from build123d import *

# Parameters (mm, degrees)
F0_R     = 15
F1_DEPTH = 25
F2_START = 25
F0_R_2   = 3
F2_DEPTH = 10
F3_R     = 10.8639610307
F4_R     = 5


with BuildPart() as f1:
    # F0 (on Top) → F1 (new body)
    with BuildSketch(Plane.XY):
        Circle(F0_R)
        Polygon((12.5, 0), (6.25, -10.8253175473), (-6.25, -10.8253175473), (-12.5, 0), (-6.25, 10.8253175473), (6.25, 10.8253175473), align=None, mode=Mode.SUBTRACT)
    extrude(amount=F1_DEPTH)

    # F0 (on Top) → F2 (join)
    with BuildSketch(Plane.XY.offset(F2_START)):
        Circle(F0_R)
        Polygon((12.5, 0), (6.25, -10.8253175473), (-6.25, -10.8253175473), (-12.5, 0), (-6.25, 10.8253175473), (6.25, 10.8253175473), align=None, mode=Mode.SUBTRACT)
        Polygon((-6.25, -10.8253175473), (6.25, -10.8253175473), (12.5, 0), (6.25, 10.8253175473), (-6.25, 10.8253175473), (-12.5, 0), align=None)
        Circle(F0_R_2, mode=Mode.SUBTRACT)
    extrude(amount=F2_DEPTH)

    # F3
    f3_edges = [f1.edges().sort_by_distance(p)[0] for p in [
        (-15, 0, 35),
    ]]
    fillet(f3_edges, radius=F3_R)

    # F4
    f4_edges = [f1.edges().sort_by_distance(p)[0] for p in [
        (-3, 0, 35),
    ]]
    fillet(f4_edges, radius=F4_R)


solid = f1.part
For this review, take the finished solid that the model builds, in its own axes (mm). A direction names the side the tool comes from. Round coordinates to 2 decimals unless told otherwise and drop trailing zeros. Loops run counter-clockwise (first coordinate to the right, second up) from the corner with the lowest first, then second, coordinate; pieces in that order, holes last. Notation, with made-up numbers: (-29, 64.5) - (22, 64.5) arc R27 cw to (22, 85.5) - close; hole circle Ø9 at (26.25, 0). An arc over 180 degrees is marked (long way). One line per question, with ' | ' between items.
Q1. For line 1 along X through (y, z) = (0, 27.5); line 2 along X through (y, z) = (5.5, 15); line 3 along Y through (x, z) = (1, 20), list the stretches that pass through material, from the lowest coordinate up. Write a range as [from, to].
Taken from the geometry:
line 1: x = [-14.47, -3], [3, 14.47] | line 2: x = [-13.96, -9.32], [9.32, 13.96] | line 3: y = [-14.97, -10.83], [10.83, 14.97]
Q2. For pin 1 (10 mm diameter, centred on y = -7.5, z = 21, fed in from -X); pin 2 (11 mm diameter, centred on x = 1, y = -4, fed in from -Z); pin 3 (6 mm diameter, centred on x = -9, z = 14, fed in from +Y), all flat-tipped, find the tip position at first contact; note any pin that passes through.
Taken from the geometry:
pin 1: stops at x = -14.79 | pin 2: stops at z = 25 | pin 3: stops at y = 13.75
Q3. The part is to be moulded in two halves that separate along X. For faces 3 (the cylindrical face through (-14.985, 0.66, 11.899)), 4 (the flat face through (-9.33, -5.49, 12.32)), 5 (the flat face through (-9, -7, 0)), 6 (the flat face through (9.33, 5.49, 12.32)), say which applies: released by +X, released by -X, zero draft, split by the parting line, or undercut.
Taken from the geometry:
face 3: split by the parting line | face 4: undercut | face 5: zero draft | face 6: undercut
Q4. Tool access review of faces 1 (the flat face through (9.419, -5.337, 12.325)), 2 (the cylindrical face through (2.86, 0.9, 26.75)): name each direction out of +Z, -Z, +X, -X, +Y, -Y from which nothing blocks a thin tool from reaching the whole face with its end or side.
Taken from the geometry:
face 1: -Z | face 2: +Z, -Z
Q5. Take a section at A-A (z = 20). Give the boundary of the cut face in (x, y).
Taken from the geometry:
outline: circle Ø30 at (0, 0); hole (-12.5, 0) - (-6.25, -10.83) - (6.25, -10.83) - (12.5, 0) - (6.25, 10.83) - (-6.25, 10.83) - close
